from build123d import *

# Parameters (mm, degrees)
SKETCH1_W           = 20
SKETCH1_H           = 40
BOSS_EXTRUDE1_DEPTH = 36
SKETCH2_W           = 20
SKETCH2_H           = 7
BOSS_EXTRUDE5_DEPTH = 3


with BuildPart() as part:
    # Sketch1 → Boss-Extrude1 (new body)
    with BuildSketch(Plane.XY):
        Rectangle(SKETCH1_W, SKETCH1_H)
    extrude(amount=BOSS_EXTRUDE1_DEPTH)

    # Sketch2 → Boss-Extrude5 (add)
    with BuildSketch(Plane.XY.offset(36)):
        with Locations((0, 23.5)):
            Rectangle(SKETCH2_W, SKETCH2_H)
        with Locations((0, -23.5)):
            Rectangle(SKETCH2_W, SKETCH2_H)
    extrude(amount=-BOSS_EXTRUDE5_DEPTH)


solid = part.part
The model under review builds one solid part; all positions refer to its coordinate system, in mm. A direction names the side the tool comes from. Give positions to 0.01 mm unless a question says otherwise; leave off trailing zeros. Order: outer loops, then holes, each group sorted by start corner. A loop starts at its lowest first (then second) coordinate and runs counter-clockwise, first axis right, second up. Notation, with made-up numbers: M -24.5,50.5 L 25.5,50.5 A16 ccw 25.5,55.5 Z; hole C 81.25,8.25 d9. An arc over 180 degrees is marked long. One line per question, with ' | ' between items. Start each with the question number.
1) Clearance check with flat-ended pins moving along their axes: P1, Ø6, axis at x = 3.5, z = 13, coming from the +Y side; P2, Ø2, axis at x = -3.5, y = -23, coming from the -Z side. State where each tip first meets the part, or that it passes through.
2) Wall thickness on L1, parallel to Y at x = -1, z = 31; L2, parallel to Z at x = 9, y = 24: over which ranges is each line inside the solid? List them lowest first. Write a range as from..to.
3) For faces 1 (the face through (0, -23, 33)), 2 (the face through (0, 20, 16)), 3 (the face through (0, 0, 0)), list the 3-axis set-ups (+Z, -Z, +X, -X, +Y, -Y) from which the entire face can be reached by the end or side of a thin tool; tool diameter is ignored.
4) Consider section A-A, the plane x = 4. Give the boundary of the cut face in (y, z).
5) Consider section B-B, the plane z = 32. Give the boundary of the cut face in (x, y).
Found:
1) P1: stops at y = 20 | P2: stops at z = 33
2) L1: y = -20..20 | L2: z = 33..36
3) face 1: -Z, +X, -X, -Y | face 2: -Z, +X, -X, +Y | face 3: -Z, +X, -X, +Y, -Y
4) outline: M -27,33 L -20,33 L -20,0 L 20,0 L 20,33 L 27,33 L 27,36 L -27,36 Z
5) outline: M -10,-20 L 10,-20 L 10,20 L -10,20 Z
